```python
from build123d import *

# Parameters (mm, degrees)
F1_DEPTH = 30
F4_W     = 2.5
F4_H     = 26
F6_R     = 1.5


with BuildPart() as f1:
    # F0 (on Top) → F1 (new body)
    with BuildSketch(Plane.XY):
        with BuildLine():
            Line((15, 20), (-15, 20))
            Line((-15, 20), (-18, 20))
            ThreePointArc((-18, 20), (-19.414214, 19.414214), (-20, 18))
            Line((-20, 18), (-20, 15))
            Line((-20, 15), (-20, -15))
            ThreePointArc((-20, -15), (-18.535534, -18.535534), (-15, -20))
            ThreePointArc((-15, -20), (-11.464466, -18.535534), (-10, -15))
            Line((-10, -15), (-10, 9.5))
            ThreePointArc((-10, 9.5), (-10.353553, 10.353553), (-9.5, 10))
            Line((-9.5, 10), (15, 10))
            ThreePointArc((15, 10), (18.535534, 11.464466), (20, 15))
            ThreePointArc((20, 15), (18.535534, 18.535534), (15, 20))
        make_face()
    extrude(amount=F1_DEPTH)

    # F5: sweep along a path in F2
    with BuildLine(Plane.XY.offset(30)) as f5_path:
        ThreePointArc((-3, 20), (-15.020815, 15.020815), (-20, 3))
    # F4 (on face) → F5 (sweep, cut)
    with BuildSketch(Plane(origin=(0, 3, 0), x_dir=(-1, 0, 0), z_dir=(0, 1, 0))):
        with Locations((21.25, 15)):
            Rectangle(F4_W, F4_H)
    sweep(path=f5_path.line, mode=Mode.SUBTRACT)

    # F6
    f6_edges = [f1.edges().sort_by_distance(p)[0] for p in [
        (-10, 9.5, 15),
        (-9.5, 10, 15),
    ]]
    fillet(f6_edges, radius=F6_R)


solid = f1.part
```
CAD build for the part. Positions are in the model's coordinates, mm. A direction names the side the tool comes from. Round coordinates to 2 decimals unless told otherwise and drop trailing zeros. Order: outer loops, then holes, each group sorted by start corner. A loop starts at its lowest first (then second) coordinate and runs counter-clockwise, first axis right, second up.
Item 1: Tool access for faces 1 (the face through (3, 10, 15)), 2 (the face through (-15.1, 15.2, 2)), 3 (the face through (-10.094, 9.2, 15.21)): list every direction of +Z, -Z, +X, -X, +Y, -Y with a clear straight run to the whole face (end or side of a thin tool).
Item 2: Saw through at A-A on z = 22. Write the cut outline in (x, y) (3 decimals), then the cut area to 3 significant figures.
Item 3: Pin check, flat tips, straight feed: pin 1 (12 mm diameter, centred on x = 0, z = 14, fed in from -Y); pin 2 (13.5 mm diameter, centred on x = -14.5, y = 9.5, fed in from -Z); pin 3 (5 mm diameter, centred on y = -2.5, z = 3.5, fed in from +X). Stop position of each tip, or through.
Item 4: Mould opens along X. For faces 4 (the face through (-9, 14, 30)), 5 (the face through (-10, -3, 15)), 6 (the face through (-9.215, 10.1, 15.21)) say: pulls with the +X half, pulls with the -X half, needs draft (parallel to the pull), parting line crosses it, or undercut.
Item 5: Probe line 1 along X through (y, z) = (0, 7.5); line 2 along Y through (x, z) = (4, 27.25); line 3 along X through (y, z) = (11, 10.25). List the from-to ranges inside material, lowest first.
Item 6: Saw through at D-D on y = -5. Write the cut outline in (x, z), then the cut area to 3 significant figures.
Item 7: Saw through at B-B on x = -14. Write the cut outline in (y, z), then the cut area to 3 significant figures.
Item 8: Saw through at C-C on x = -6.5. Write the cut outline in (y, z), then the cut area to 3 significant figures.
Reported:
1. face 1: +Z, -Z, +X, -Y
1. face 2: none
1. face 3: +Z, -Z, +X
2. outline: (-20, -15) arc R5 ccw to (-10, -15) - (-10, 8.677) arc R1.5 ccw to (-10.375, 9.669) arc R0.5 cw to (-9.669, 10.375) arc R1.5 ccw to (-8.677, 10) - (15, 10) arc R5 ccw to (15, 20) - (-3, 20) arc R17 ccw to (-20, 3) - close; (-20, 12.552) arc R19.5 cw to (-12.552, 20) - (-18, 20) arc R2 ccw to (-20, 18) - close
2. area: 638 mm2
3. pin 1: stops at y = 10
3. pin 2: stops at z = 0
3. pin 3: stops at x = -10
4. face 4: needs draft
4. face 5: pulls with the +X half
4. face 6: undercut
5. line 1: x = -20 to -10
5. line 2: y = 10 to 20
5. line 3: x = -18 to 18
6. outline: (-20, 0) - (-10, 0) - (-10, 30) - (-20, 30) - close
6. area: 300 mm2
7. outline: (-19.9, 0) - (20, 0) - (20, 30) - (-19.9, 30) - close; hole (15.96, 2) - (19.1, 2) - (19.1, 28) - (15.96, 28) - close
7. area: 1,120 mm2
8. outline: (10, 0) - (20, 0) - (20, 2) - (19.64, 2) - (19.64, 28) - (20, 28) - (20, 30) - (10, 30) - close
8. area: 291 mm2
